from build123d import *

# Parameters (mm, degrees)
BOSS_EXTRUDE1_DEPTH = 10
CUT_EXTRUDE1_DEPTH  = 11
SKETCH3_R           = 1.75
CUT_EXTRUDE2_DEPTH  = 91.9


with BuildPart() as part:
    # Sketch1 → Boss-Extrude1 (new body)
    with BuildSketch(Plane.XY):
        Polygon((0, 0), (0, 5), (-10, 5), (-10, 10), (0, 10), (0, 91), (-10, 91), (-10, 96), (10, 96), (10, 0), align=None)
    extrude(amount=-BOSS_EXTRUDE1_DEPTH)

    # Sketch2 → Cut-Extrude1 (cut, through all)
    with BuildSketch(Plane.XY):
        Polygon((-10, 10), (-10, 5), (0, 5), (0, 0), (0.1, 0), (0.1, 5.1), (-9.9, 5.1), (-9.9, 10), align=None)
        Polygon((-10, 96), (-10, 91), (0, 91), (0, 85.9), (0.1, 85.9), (0.1, 91.1), (-9.9, 91.1), (-9.9, 96), align=None)
    extrude(amount=-CUT_EXTRUDE1_DEPTH, mode=Mode.SUBTRACT)

    # Sketch3 → Cut-Extrude2 (cut, through all)
    with BuildSketch(Plane.XZ.offset(-5.1)):
        with Locations((-5, -5)):
            Circle(SKETCH3_R)
    extrude(amount=-CUT_EXTRUDE2_DEPTH, mode=Mode.SUBTRACT)


solid = part.part
Build history of the part. All positions in model axes, mm. A direction names the side the tool comes from. Coordinates: 2 decimals unless noted, no trailing zeros. Write each loop counter-clockwise with the first axis right and the second up, starting at its lowest first coordinate (ties: lowest second). Pieces come first, ordered by that corner, then holes. Notation, with made-up numbers: (26.25, -35.5) -> (42.25, -35.5) arc R17 ccw to (42.25, -26.5) -> close; hole circle Ø3 at (47.25, 81). An arc over 180 degrees is marked (long way). Use CSV: the item, a comma, the result in double quotes. Start each with the question number.
Q1. Cut at D-D, the plane z = -1.25. List the corners of the cut face in (x, y), then the cut area to 3 significant figures.
Q2. Cut at A-A, the plane z = -5. List the corners of the cut face in (x, y).
Q3. Drill centre lines: probe 1 along Z at (x, y) = (-5, 94.8); probe 2 along Y at (x, z) = (-6.25, -8.25); probe 3 along X at (y, z) = (87, -3.5). Where is each one in solid material? Low to high.
Q4. Cut at B-B, the plane x = -5. List the corners of the cut face in (y, z), then the cut area to 3 significant figures.
Q5. 3-axis set-ups, long thin cutter, end or side, ignore diameter. For faces 1 (the flat face through (-9.9, 8, -5)), 2 (the flat face through (-3, 91.1, -5)), 3 (the flat face through (0.1, 3, -5)): which of +Z, -Z, +X, -X, +Y, -Y reach the whole face in a straight line?
Q6. Flat gauge pins, fed straight in: pin 1 Ø5.5 at (y, z) = (1.5, -5.5) entering from -X; pin 2 Ø5 at (x, z) = (-4.5, -4) entering from -Y; pin 3 Ø6 at (y, z) = (19.5, -5.5) entering from -X. Where does each tip first touch, or does it go through?
Q7. Cut at C-C, the plane x = -1. List the corners of the cut face in (y, z).
Q8. Pull direction X, two halves, no side cores. Call faces 4 (the flat face through (5, 0, -5)), 5 (the cylindrical face through (-5.38, 93.52, -6.71)), 6 (the flat face through (0.1, 88, -5)): released by +X, released by -X, zero draft, split by the parting line, or undercut.
Checked values:
1,outline,"(-9.9, 5.1) -> (0.1, 5.1) -> (0.1, 0) -> (10, 0) -> (10, 96) -> (-9.9, 96) -> (-9.9, 91.1) -> (0.1, 91.1) -> (0.1, 85.9) -> (0, 85.9) -> (0, 10) -> (-9.9, 10) -> close"
1,area,"1,060 mm²"
2,outline,"(-9.9, 5.1) -> (-6.75, 5.1) -> (-6.75, 10) -> (-9.9, 10) -> close; (-9.9, 91.1) -> (-6.75, 91.1) -> (-6.75, 96) -> (-9.9, 96) -> close; (-3.25, 5.1) -> (0.1, 5.1) -> (0.1, 0) -> (10, 0) -> (10, 96) -> (-3.25, 96) -> (-3.25, 91.1) -> (0.1, 91.1) -> (0.1, 85.9) -> (0, 85.9) -> (0, 10) -> (-3.25, 10) -> close"
3,probe 1,"z = -10 to -6.75, -3.25 to 0"
3,probe 2,"y = 5.1 to 10, 91.1 to 96"
3,probe 3,"x = 0.1 to 10"
4,outline,"(5.1, -10) -> (10, -10) -> (10, -6.75) -> (5.1, -6.75) -> close; (5.1, -3.25) -> (10, -3.25) -> (10, 0) -> (5.1, 0) -> close; (91.1, -10) -> (96, -10) -> (96, -6.75) -> (91.1, -6.75) -> close; (91.1, -3.25) -> (96, -3.25) -> (96, 0) -> (91.1, 0) -> close"
4,area,"63.7 mm²"
5,face 1,"+Z, -Z, -X, +Y, -Y"
5,face 2,"+Z, -Z, -X"
5,face 3,"+Z, -Z, -X, -Y"
6,pin 1,"stops at x = 0.1"
6,pin 2,"stops at y = 5.1"
6,pin 3,"stops at x = 0"
7,outline,"(5.1, -10) -> (10, -10) -> (10, 0) -> (5.1, 0) -> close; (91.1, -10) -> (96, -10) -> (96, 0) -> (91.1, 0) -> close"
8,face 4,"zero draft"
8,face 5,"undercut"
8,face 6,"released by -X"
